Geometry check sheet. Reference: the model listing, model coordinates, mm. Face numbers are marked on the shaded views. A direction names the side the tool comes from. Round coordinates to 2 decimals unless told otherwise and drop trailing zeros. Write each loop counter-clockwise with the first axis right and the second up, starting at its lowest first coordinate (ties: lowest second). Pieces come first, ordered by that corner, then holes. Notation, with made-up numbers: M 3,37.25 L 10,37.25 A33 ccw 10,67.25 Z; hole C 32.25,43.25 d9. An arc over 180 degrees is marked long. Answer in a Markdown table with one row per item. Add a question column.
from build123d import *

# Parameters (mm, degrees)
SKETCH_4_W                = 34.4
SKETCH_4_H                = 57.6
EXTRUDE_3_DEPTH           = 90
SHELL_2_OUTLINE_R         = 62.2
SHELL_2_OUTLINE_R_2       = 19
SHELL_2_DEPTH             = 177
SHELL_START               = 125.4
SHELL_2_2_DEPTH           = 51.6
SHELL_2_3_OUTLINE_R       = 19
SHELL_2_3_DEPTH           = 36
EXTRUDE_4_DEPTH           = 3
CUT_EXTRUDE_START         = -3
SKETCH_9_R                = 16
CUT_EXTRUDE_1_DEPTH       = 3
SKETCH_10_R               = 19
CUT_EXTRUDE_2_DEPTH       = 3
CUT_EXTRUDE_START_2       = -2
CUT_EXTRUDE_3_OUTLINE_R   = 65.2
CUT_EXTRUDE_3_OUTLINE_R_2 = 63.2
CUT_EXTRUDE_3_DEPTH       = 2


# Read off the part's stored shape, not the designer's step: 쉘2, 컷-돌출3
with BuildPart() as part:
    # 스케치3 → 회전1 (revolve)
    with BuildSketch(Plane.XY, mode=Mode.PRIVATE) as revolve_1_sk:
        Polygon((0, 36), (16, 36), (16, 180), (65.2, 180), (65.2, 0), (0, 0), align=None)
    revolve(revolve_1_sk.sketch.rotate(Axis((0, 0, 0), (0, 1, 0)), 90), axis=Axis((0, 0, 0), (0, 1, 0)))

    # 스케치4 → 보스-돌출3 (add)
    with BuildSketch(Plane.XY):
        with Locations((-48, 151.2)):
            Rectangle(SKETCH_4_W, SKETCH_4_H)
    extrude(amount=EXTRUDE_3_DEPTH)

    # 쉘2 outline → 쉘2 (cut)
    with BuildSketch(Plane(origin=(0, 0, 0), x_dir=(1, 0, 0), z_dir=(0, 1, 0))):
        Circle(SHELL_2_OUTLINE_R)
        Circle(SHELL_2_OUTLINE_R_2, mode=Mode.SUBTRACT)
    extrude(amount=SHELL_2_DEPTH, mode=Mode.SUBTRACT)

    # Shell 2 2 outline → Shell 2 2 (cut)
    with BuildSketch(Plane(origin=(0, 0, 0), x_dir=(1, 0, 0), z_dir=(0, 1, 0)).offset(SHELL_START)):
        with BuildLine():
            ThreePointArc((-33.8, -52.214940391), (-54.640644213, -29.719353963), (-62.2, 0))
            Line((-62.2, 0), (-62.2, -90))
            Line((-62.2, -90), (-33.8, -90))
            Line((-33.8, -90), (-33.8, -52.214940391))
        make_face()
    extrude(amount=SHELL_2_2_DEPTH, mode=Mode.SUBTRACT)

    # Shell 2 3 outline → Shell 2 3 (cut)
    with BuildSketch(Plane(origin=(0, 0, 0), x_dir=(1, 0, 0), z_dir=(0, 1, 0))):
        Circle(SHELL_2_3_OUTLINE_R)
    extrude(amount=SHELL_2_3_DEPTH, mode=Mode.SUBTRACT)

    # 스케치8 → 보스-돌출4 (add)
    with BuildSketch(Plane(origin=(0, 180, 0), x_dir=(1, 0, 0), z_dir=(0, 1, 0))):
        with BuildLine():
            Line((-30.8, -90), (-30.8, -57.466511987))
            ThreePointArc((-30.8, -57.466511987), (55.942827959, 33.487908266), (-65.2, 0))
            Line((-65.2, 0), (-65.2, -90))
            Line((-65.2, -90), (-30.8, -90))
        make_face()
    extrude(amount=EXTRUDE_4_DEPTH)

    # 스케치9 → 컷-돌출1 (cut)
    with BuildSketch(Plane.XZ.offset(-180).offset(CUT_EXTRUDE_START)):
        with Locations(Location((0, 0, 0), (0, 0, 270))):
            Circle(SKETCH_9_R)
    extrude(amount=CUT_EXTRUDE_1_DEPTH, mode=Mode.SUBTRACT)

    # 스케치10 → 컷-돌출2 (cut)
    with BuildSketch(Plane(origin=(0, 183, 0), x_dir=(1, 0, 0), z_dir=(0, 1, 0)).offset(CUT_EXTRUDE_START)):
        with Locations(Location((0, 0, 0), (0, 0, 270))):
            Circle(SKETCH_10_R)
    extrude(amount=CUT_EXTRUDE_2_DEPTH, mode=Mode.SUBTRACT)

    # 컷-돌출3 outline → 컷-돌출3 (cut)
    with BuildSketch(Plane.XZ.offset(CUT_EXTRUDE_START_2)):
        Circle(CUT_EXTRUDE_3_OUTLINE_R)
        Circle(CUT_EXTRUDE_3_OUTLINE_R_2, mode=Mode.SUBTRACT)
    extrude(amount=CUT_EXTRUDE_3_DEPTH, mode=Mode.SUBTRACT)


solid = part.part
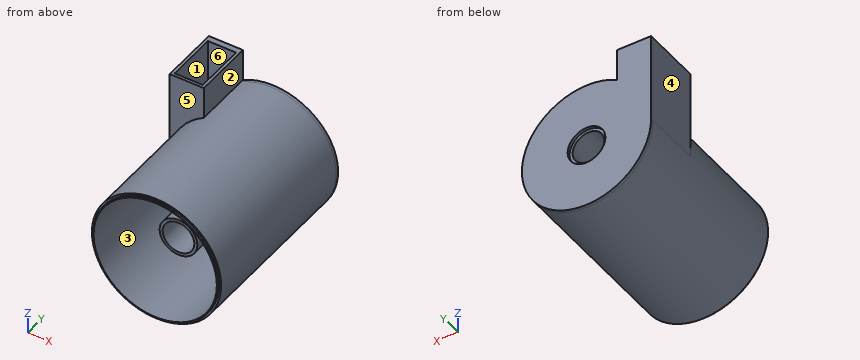
Item 1: Scan lines: probe 1 along X at (y, z) = (69, 0); probe 2 along X at (y, z) = (182.15, 0); probe 3 along X at (y, z) = (79.5, -7). Record each from-to range of solid material in increasing order. Write a range as from..to.
Item 2: Mould release check, pull along X, two halves, no side actions. Record for the marked faces 4, 5 and 6: +X half, -X half, draft (parallel to the pull), parting line (faces both ways), or undercut.
Item 3: Section check C-C, the plane y = 68. Record the boundary of the cut face in (x, z).
Item 4: Section check B-B, the plane x = 0. Record the boundary of the cut face in (y, z).
Item 5: Gauge pin test, flat ends, axial feed: pin 1 Ø2 at (y, z) = (44, 18.5) entering from -X; pin 2 Ø8 at (y, z) = (75, 11) entering from +X; pin 3 Ø15.5 at (y, z) = (161.5, 53) entering from +X; pin 4 Ø19 at (x, z) = (3.5, -1.5) entering from +Y. Record the tip position at first contact, or that the pin passes through.
Item 6: Section check D-D, the plane z = -33.5. Record the boundary of the cut face in (x, y).
Item 7: Access from +Z, -Z, +X, -X, +Y, -Y to the whole of each face (thin tool, end or side, straight path). Record for the marked faces 1, 2 and 3.
Item 8: Section check A-A, the plane y = 166. Record the boundary of the cut face in (x, z), and give its area (3 significant figures).
Result sheet:
| question | item | result |
|---|---|---|
| 1 | probe 1 | x = -65.2..-62.2, -19..-16, 16..19, 62.2..65.2 |
| 1 | probe 2 | x = -65.2..-19, 19..65.2 |
| 1 | probe 3 | x = -64.82..-61.8, -17.66..-14.39, 14.39..17.66, 61.8..64.82 |
| 2 | face 4 | -X half |
| 2 | face 5 | draft |
| 2 | face 6 | undercut |
| 3 | outline | C 0,0 d130.4; C 0,0 d38; hole C 0,0 d124.4; hole C 0,0 d32 |
| 4 | outline | M 0,-63.2 L 2,-63.2 L 2,-65.2 L 183,-65.2 L 183,-19 L 180,-19 L 180,-16 L 36,-16 L 36,-19 L 177,-19 L 177,-62.2 L 0,-62.2 Z; M 0,62.2 L 177,62.2 L 177,19 L 36,19 L 36,16 L 180,16 L 180,19 L 183,19 L 183,65.2 L 2,65.2 L 2,63.2 L 0,63.2 Z |
| 5 | pin 1 | stops at x = -62.81 |
| 5 | pin 2 | stops at x = 64.82 |
| 5 | pin 3 | stops at x = 46.94 |
| 5 | pin 4 | passes through |
| 6 | outline | M -55.94,2 L -53.59,2 L -53.59,0 L -52.41,0 L -52.41,177 L 52.41,177 L 52.41,0 L 53.59,0 L 53.59,2 L 55.94,2 L 55.94,183 L -55.94,183 Z |
| 7 | face 1 | +Z |
| 7 | face 2 | +Z, +Y, -Y |
| 7 | face 3 | -Y |
| 8 | outline | M -65.2,0 A65.2 ccw long -30.8,57.47 L -30.8,90 L -33.8,90 L -33.8,52.21 A62.2 cw long -62.2,0 L -62.2,90 L -65.2,90 Z; C 0,0 d38; hole C 0,0 d32 |
| 8 | area | 1,710 mm^2 |
